```python
from build123d import *

# Parameters (mm, degrees)
BOSS_EXTRUDE1_DEPTH        = 365.125
F_10_32_TAPPED_HOLE1_D     = 4.0386
F_10_32_TAPPED_HOLE1_DEPTH = 12.0396
F_10_32_TAPPED_HOLE1_TIP   = 1.213317848
F_10_32_TAPPED_HOLE2_D     = 4.0386
F_10_32_TAPPED_HOLE2_DEPTH = 12.0396
F_10_32_TAPPED_HOLE2_TIP   = 1.213317848
SKETCH6_W                  = 2.032
SKETCH6_H                  = 2.353948419


with BuildPart() as part:
    # Sketch1 → Boss-Extrude1 (new body)
    with BuildSketch(Plane(origin=(0, 0, 0), x_dir=(0, 0, -1), z_dir=(1, 0, 0))):
        Polygon((0, 7.332348419), (-6.35, 3.666174209), (-6.35, -3.666174209), (0, -7.332348419), (6.35, -3.666174209), (6.35, 3.666174209), align=None)
    extrude(amount=BOSS_EXTRUDE1_DEPTH)

    # #10-32 Tapped Hole1
    with Locations(Plane(origin=(365.125, 0, 0), x_dir=(0, 0, -1), z_dir=(1, 0, 0))):
        with Locations((0, 0)):
            Hole(F_10_32_TAPPED_HOLE1_D / 2, depth=F_10_32_TAPPED_HOLE1_DEPTH)
            with Locations((0, 0, -(F_10_32_TAPPED_HOLE1_DEPTH + F_10_32_TAPPED_HOLE1_TIP / 2))):  # 118° drill point
                Cone(0, F_10_32_TAPPED_HOLE1_D / 2, F_10_32_TAPPED_HOLE1_TIP, mode=Mode.SUBTRACT)

    # #10-32 Tapped Hole2
    with Locations(Plane.ZY):
        with Locations((0, 0)):
            Hole(F_10_32_TAPPED_HOLE2_D / 2, depth=F_10_32_TAPPED_HOLE2_DEPTH)
            with Locations((0, 0, -(F_10_32_TAPPED_HOLE2_DEPTH + F_10_32_TAPPED_HOLE2_TIP / 2))):  # 118° drill point
                Cone(0, F_10_32_TAPPED_HOLE2_D / 2, F_10_32_TAPPED_HOLE2_TIP, mode=Mode.SUBTRACT)

    # Sketch6 → Cut-Revolve1 (revolve, cut)
    with BuildSketch(Plane.XY):
        with Locations((56.134, 6.15537421)):
            Rectangle(SKETCH6_W, SKETCH6_H)
        with Locations((67.564, 6.15537421)):
            Rectangle(SKETCH6_W, SKETCH6_H)
        with Locations((297.561, 6.15537421)):
            Rectangle(SKETCH6_W, SKETCH6_H)
        with Locations((308.991, 6.15537421)):
            Rectangle(SKETCH6_W, SKETCH6_H)
    revolve(axis=Axis((0, 0, 0), (1, 0, 0)), mode=Mode.SUBTRACT)


solid = part.part
```
Build history of the part. All positions in model axes, mm. A direction names the side the tool comes from. Give positions to 0.01 mm unless a question says otherwise; leave off trailing zeros. Order: outer loops, then holes, each group sorted by start corner. A loop starts at its lowest first (then second) coordinate and runs counter-clockwise, first axis right, second up. Notation, with made-up numbers: M 84.5,-35 L 113.5,-35 A25 ccw 113.5,-18 Z; hole C 26,-29 d10. An arc over 180 degrees is marked long. Return JSON: item names as keys, results as strings.
Q1. Two-plate mould, pull along X, no slides. Class faces 1 (the face through (27, 0, 6.35)), 2 (the face through (307.975, -4.3, 2.9)): pulls with the +X half, pulls with the -X half, needs draft (parallel to the pull), parting line crosses it, or undercut.
Answer list:
{"face 1": "needs draft", "face 2": "undercut"}
Q2. 3-axis set-ups, long thin cutter, end or side, ignore diameter. For faces 3 (the face through (57.15, -4.3, 2.9)), 4 (the face through (303, 0, -6.35)): which of +Z, -Z, +X, -X, +Y, -Y reach the whole face in a straight line?
Answer list:
{"face 3": "none", "face 4": "-Z, +X, -X, +Y, -Y"}
Q3. Band-saw the part on A-A (x = 144). Give the cut face in (y, z).
Answer list:
{"outline": "M -7.33,0 L -3.67,-6.35 L 3.67,-6.35 L 7.33,0 L 3.67,6.35 L -3.67,6.35 Z"}
Q4. Flat gauge pins, fed straight in: pin 1 (6.5 mm diameter, centred on y = 0.5, z = -3, fed in from -X); pin 2 (1 mm diameter, centred on x = 213, y = 4.5, fed in from +Z); pin 3 (1.5 mm diameter, centred on x = 45, y = -5, fed in from +Z). Where does each tip first touch, or does it go through?
Answer list:
{"pin 1": "stops at x = 0", "pin 2": "stops at z = 5.77", "pin 3": "stops at z = 5.34"}
Q5. Wall check: probe 1 along X at (y, z) = (3, -5) (3 decimals); probe 2 along Y at (x, z) = (8, 0); probe 3 along Z at (x, y) = (357, 0). Give the ranges that are in metal, low to high. Write a range as from..to.
Answer list:
{"probe 1": "x = 0..55.118, 57.15..66.548, 68.58..296.545, 298.577..307.975, 310.007..365.125", "probe 2": "y = -7.33..-2.02, 2.02..7.33", "probe 3": "z = -6.35..-2.02, 2.02..6.35"}
